Source: CAD feature listing. Evaluate the final solid. Frame: model axes, mm. Face numbers are marked on the shaded views. Round coordinates to 2 decimals unless told otherwise and drop trailing zeros. Order: outer loops, then holes, each group sorted by start corner. A loop starts at its lowest first (then second) coordinate and runs counter-clockwise, first axis right, second up. Notation, with made-up numbers: (-27, 89.25) - (31, 89.25) arc R23 cw to (31, 109.25) - close; hole circle Ø4 at (0, -30). An arc over 180 degrees is marked (long way). Return JSON: item names as keys, results as strings. Group by question number.
1) Section A-A, the plane x = 30. Return loops of the section in (y, z).
2) Section B-B, the plane y = 1. Return loops of the section in (x, z), plus the area to 3 significant figures.
3) Section D-D, the plane x = -6.5. Return loops of the section in (y, z).
4) Section C-C, the plane x = 1.5. Return loops of the section in (y, z).
5) Ray query, line 1 (Y direction, x = 30, z = -10.35); line 2 (Z direction, x = 10, y = 11.75); line 3 (X direction, y = 5, z = -10). Return the intervals inside material, ascending. Write a range as from..to.
6) Mould query, pull axis Z, two halves, no side actions, for the marked faces 1, 2 and 3. Classes: pulls with the +Z half, pulls with the -Z half, needs draft (parallel to the pull), parting line crosses it, or undercut.
7) Contact query for flat-ended pins moving along their axis: P1, Ø8, axis at x = 2, z = -3.5, coming from the -Y side; P2, Ø1.8, axis at y = 8.5, z = 10.5, coming from the +X side; P3, Ø3, axis at y = 3.5, z = 4, coming from the +X side; P4, Ø4, axis at y = 10, z = 3.5, coming from the -X side. Output: stop coordinate, or through.
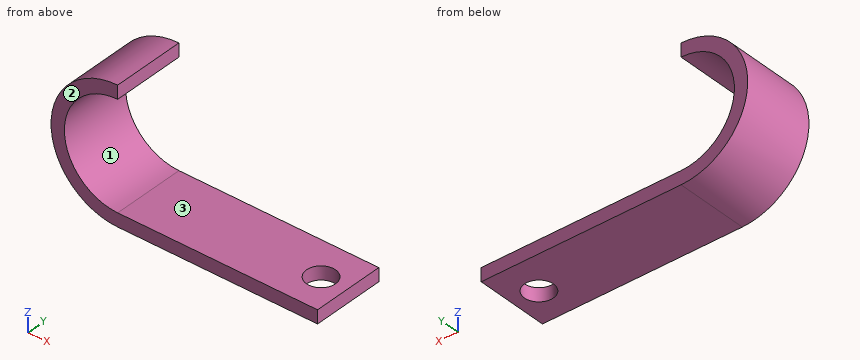
```python
from build123d import *

# Parameters (mm, degrees)
BOSS_EXTRUDE1_DEPTH = 12.6
SKETCH2_R           = 2.5
CUT_EXTRUDE1_DEPTH  = 12.6


with BuildPart() as part:
    # Sketch1 → Boss-Extrude1 (new body)
    with BuildSketch(Plane(origin=(0, 0, 0), x_dir=(1, 0, 0), z_dir=(0, 1, 0))):
        with BuildLine():
            Line((0, 11.5), (11.5, 11.5))
            Line((11.5, 11.5), (34.5, 11.5))
            Line((34.5, 11.5), (34.5, 9.2))
            Line((34.5, 9.2), (0, 9.2))
            ThreePointArc((0, 9.2), (-9.2, 0), (0, -9.2))
            Line((0, -9.2), (0, -11.5))
            ThreePointArc((0, -11.5), (-11.5, 0), (0, 11.5))
        make_face()
    extrude(amount=BOSS_EXTRUDE1_DEPTH)

    # Sketch2 → Cut-Extrude1 (cut)
    with BuildSketch(Plane.XY.offset(-9.2)):
        with Locations((30, 6.079989629)):
            Circle(SKETCH2_R)
    extrude(amount=-CUT_EXTRUDE1_DEPTH, mode=Mode.SUBTRACT)


solid = part.part
```
Geometry check:
{
 "1": {"outline": "(0, -11.5) - (3.58, -11.5) - (3.58, -9.2) - (0, -9.2) - close; (8.58, -11.5) - (12.6, -11.5) - (12.6, -9.2) - (8.58, -9.2) - close"},
 "2": {"outline": "(0, -11.5) - (34.5, -11.5) - (34.5, -9.2) - (0, -9.2) arc R9.2 cw to (0, 9.2) - (0, 11.5) arc R11.5 ccw to start", "area": "154 mm2"},
 "3": {"outline": "(0, -9.49) - (12.6, -9.49) - (12.6, -6.51) - (0, -6.51) - close; (0, 6.51) - (12.6, 6.51) - (12.6, 9.49) - (0, 9.49) - close"},
 "4": {"outline": "(0, -11.5) - (12.6, -11.5) - (12.6, -9.2) - (0, -9.2) - close"},
 "5": {"line 1": "0..3.58, 8.58..12.6", "line 2": "-11.5..-9.2", "line 3": "-5.68..27.75, 32.25..34.5"},
 "6": {"face 1": "undercut", "face 2": "needs draft", "face 3": "pulls with the +Z half"},
 "7": {"P1": "through", "P2": "x = 0", "P3": "x = -7.37", "P4": "x = -11.4"}
}
